Here's how the part is built. I have some questions about the finished solid (model axes, mm). Face numbers are marked on the shaded views. A direction names the side the tool comes from. Give positions to 0.01 mm unless a question says otherwise; leave off trailing zeros. Loops run counter-clockwise (first coordinate to the right, second up) from the corner with the lowest first, then second, coordinate; pieces in that order, holes last. Notation, with made-up numbers: (-30.5, -4) - (-21.5, -4) arc R13 cw to (-21.5, 15) - close; hole circle Ø2 at (57, 34.5). An arc over 180 degrees is marked (long way). One line per item, written item: value. Start each with the question number.
```python
from build123d import *

# Parameters (mm, degrees)
SZKIC4_W                   = 14
SZKIC4_H                   = 0.05
SFAZOWANIE1_SIZE           = 0.35
ZAOKR_GLENIE1_R            = 0.35
WYTNIJ_WYCI_GNI_CIE1_DEPTH = 1


with BuildPart() as part:
    # Szkic1 → Obrót1 (revolve)
    with BuildSketch(Plane.XY):
        Polygon((0, 0), (0, 3.5), (-2.5, 3.5), (-2.5, 2), (-18.5, 2), (-18.5, 0), align=None)
    revolve(axis=Axis((-123.158940217, 0, 0), (1, 0, 0)))

    # Szkic4 → Wycięcie-obrót1 (revolve, cut)
    with BuildSketch(Plane(origin=(0, 0, 0), x_dir=(1, 0, 0), z_dir=(0, 1, 0))):
        with Locations((-11.5, -1.975)):
            Rectangle(SZKIC4_W, SZKIC4_H)
    revolve(axis=Axis((0, 0, 0), (-1, 0, 0)), mode=Mode.SUBTRACT)

    # Sfazowanie1
    sfazowanie1_edges = [part.edges().sort_by_distance(p)[0] for p in [
        (-18.5, 0, -1.95),
    ]]
    chamfer(sfazowanie1_edges, length=SFAZOWANIE1_SIZE)

    # Zaokrąglenie1
    zaokr_glenie1_edges = [part.edges().sort_by_distance(p)[0] for p in [
        (0, -3.5, 0),
    ]]
    fillet(zaokr_glenie1_edges, radius=ZAOKR_GLENIE1_R)

    # Szkic2 → Wytnij-wyciągnięcie1 (cut)
    with BuildSketch(Plane(origin=(0, 0, 0), x_dir=(0, 0, -1), z_dir=(1, 0, 0))):
        Polygon((1.154700538, 0), (0.577350269, 1), (-0.577350269, 1), (-1.154700538, 0), (-0.577350269, -1), (0.577350269, -1), align=None)
    extrude(amount=-WYTNIJ_WYCI_GNI_CIE1_DEPTH, mode=Mode.SUBTRACT)


solid = part.part
```
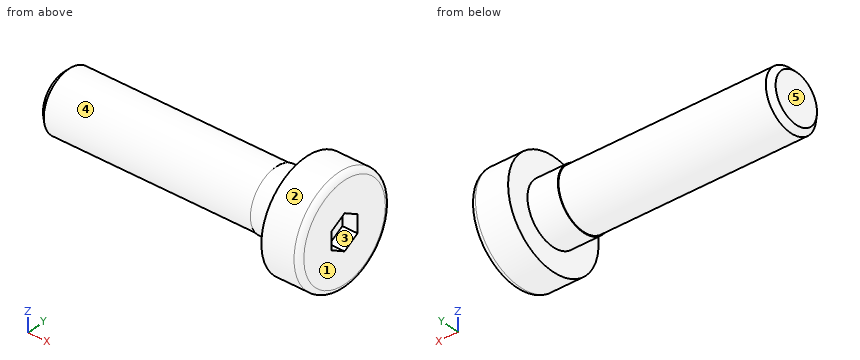
(1) If we section it at B-B on x = -13.75: List the corners of the cut face in (y, z) for me, plus the area to 3 significant figures.
(2) If we section it at A-A on z = 0: List the corners of the cut face in (x, y) for me.
(3) Will these pins go through, and if not, where does the flat tip stop? pin 1 (1.5 mm diameter, centred on x = -2, y = 2, fed in from -Z); pin 2 (2 mm diameter, centred on x = -8.5, z = 0, fed in from +Y); pin 3 (2 mm diameter, centred on x = -16.5, y = 0, fed in from +Z).
(4) If we section it at C-C on x = -4: List the corners of the cut face in (y, z) for me.
(5) For the marked faces 4 and 5, which set-ups out of +Z, -Z, +X, -X, +Y, -Y let a thin tool reach every point of the face, with its end or its side?
(6) Please list where these lines run through material, in increasing order: probe 1 along X at (y, z) = (-2, -2.5); probe 2 along X at (y, z) = (0, -0.75); probe 3 along Y at (x, z) = (-8.5, -0.25). Write a range as from..to.
(7) If we mould it in two halves opening along Z, with no side actions, what happens to the marked faces 1, 2 and 3? For each: pulls with the +Z half, pulls with the -Z half, needs draft (parallel to the pull), parting line crosses it, or undercut.
Found:
1. outline: circle Ø3.9 at (0, 0)
1. area: 11.9 mm^2
2. outline: (-18.5, -1.6) - (-18.15, -1.95) - (-4.5, -1.95) - (-4.5, -2) - (-2.5, -2) - (-2.5, -3.5) - (-0.35, -3.5) arc R0.35 ccw to (0, -3.15) - (0, -1) - (-1, -1) - (-1, 1) - (0, 1) - (0, 3.15) arc R0.35 ccw to (-0.35, 3.5) - (-2.5, 3.5) - (-2.5, 2) - (-4.5, 2) - (-4.5, 1.95) - (-18.15, 1.95) - (-18.5, 1.6) - close
3. pin 1: z = -3.27
3. pin 2: y = 1.95
3. pin 3: z = 1.95
4. outline: circle Ø4 at (0, 0)
5. face 4: -X
5. face 5: +Z, -Z, -X, +Y, -Y
6. probe 1: -2.5..0
6. probe 2: -18.5..-1
6. probe 3: -1.93..1.93
7. face 1: needs draft
7. face 2: parting line crosses it
7. face 3: undercut
